Check sheet for the modelled part. Datum: model origin and axes. Units: mm. A direction names the side the tool comes from. Round coordinates to 2 decimals unless told otherwise and drop trailing zeros. Write each loop counter-clockwise with the first axis right and the second up, starting at its lowest first coordinate (ties: lowest second). Pieces come first, ordered by that corner, then holes. Notation, with made-up numbers: M 56,9 L 90,9 A28 cw 90,45 Z; hole C 8.5,55.5 d1. An arc over 180 degrees is marked long. Put each result on its own line as item: value.
Autodesk Inventor part; units mm, degrees
ref_plane "YZ Plane" through (0, 0, 0) normal (1, 0, 0) x (0, 1, 0)
ref_plane "XZ Plane" through (0, 0, 0) normal (0, 1, 0) x (-1, 0, 0)
ref_plane "XY Plane" through (0, 0, 0) normal (0, 0, 1) x (1, 0, 0)
sketch "Sketch1" plane through (0, 0, 0) normal (0, 1, 0) x (-1, 0, 0)
  line L0 (15, 0) -> (-15, 0) construction
  line L1 (15, 5) -> (-15, 5)
  line L2 (-15, -5) -> (15, -5)
  arc A0 (15, -5) -> (15, 5) centre (15, 0) ccw
  arc A1 (-15, 5) -> (-15, -5) centre (-15, 0) ccw
  point P0 (0, 0)
  dimension "d0" = 15
  dimension "d1" = 10
extrude "Extrusion1" add sketch "Sketch1" along normal blind 2
sketch "Sketch2" plane through (0, 2, 0) normal (0, 1, 0) x (1, 0, 0)
  circle A0 centre (0, 0) radius 3.5
  dimension "d4" = 7
extrude "Extrusion2" add sketch "Sketch2" along normal blind 3
sketch "Sketch3" plane through (0, 5, 0) normal (0, 1, 0) x (1, 0, 0)
  circle A0 centre (0, 0) radius 2.5
  dimension "d7" = 5
extrude "Extrusion3" cut sketch "Sketch3" against normal blind 4
properties part number "tang"
1. Depth check by flat-ended pin: pin 1 Ø2 at (x, z) = (-8.5, 2.5) entering from +Y. Enter the tip coordinate at first touch or a pass-through.
Computed values:
pin 1: stops at y = 2
2. Scan lines: probe 1 along Z at (x, y) = (0, 3.85); probe 2 along Z at (x, y) = (0, 1.9). Record each from-to range of solid material in increasing order.
Computed values:
probe 1: z = -3.5 to -2.5, 2.5 to 3.5
probe 2: z = -5 to -2.5, 2.5 to 5
3. Cross-section at C-C (y = 4.3). Enter the section's corners in (x, z).
Computed values:
outline: C 0,0 d7; hole C 0,0 d5
4. Access from +Z, -Z, +X, -X, +Y, -Y to the whole of each face (thin tool, end or side, straight path). Record for faces 4 (the cylindrical face through (20, 1, 0)), 5 (the cylindrical face through (3.233, 3.479, -1.341)).
Computed values:
face 4: +X, +Y, -Y
face 5: +Y
5. Cross-section at A-A (x = 0). Enter the section's corners in (y, z), then the cut area to 3 significant figures.
Computed values:
outline: M 0,-5 L 2,-5 L 2,-3.5 L 5,-3.5 L 5,-2.5 L 1,-2.5 L 1,2.5 L 5,2.5 L 5,3.5 L 2,3.5 L 2,5 L 0,5 Z
area: 21.0 mm2
6. Cross-section at B-B (z = 0). Enter the section's corners in (x, y).
Computed values:
outline: M -20,0 L 20,0 L 20,2 L 3.5,2 L 3.5,5 L 2.5,5 L 2.5,1 L -2.5,1 L -2.5,5 L -3.5,5 L -3.5,2 L -20,2 Z
7. Cross-section at D-D (z = -3). Enter the section's corners in (x, y).
Computed values:
outline: M -19,0 L 19,0 L 19,2 L 1.8,2 L 1.8,5 L -1.8,5 L -1.8,2 L -19,2 Z
8. Release check for a two-part mould opening along X. For faces 1 (the cylindrical face through (-20, 1, 0)), 2 (the flat face through (0, 1, 0)), 3 (the flat face through (0, 1, -5)) record: +X half, -X half, draft (parallel to the pull), parting line (faces both ways), or undercut.
Computed values:
face 1: -X half
face 2: undercut
face 3: draft
